from build123d import *

# Parameters (mm, degrees)
ESTRUSIONE_ESTRUSIONE1_DEPTH = 140
FORO_6_5_6_5_1_D             = 6.5
FORO_6_5_6_5_2_AT_2_COUNT    = 2
FORO_6_5_6_5_2_AT_2_PITCH    = 25
TAGLIO_ESTRUSIONE1_REACH     = 158.844
SCHIZZO8_R                   = 1.75
TAGLIO_ESTRUSIONE2_REACH     = 158.844
SCHIZZO9_R                   = 1.75
SCHIZZO9_R_2                 = 7
TAGLIO_ESTRUSIONE4_REACH     = 158.844
SCHIZZO11_R                  = 4
SCHIZZO11_R_2                = 1.75
SMUSSO1_SIZE                 = 3


with BuildPart() as part:
    # Schizzo1 → Estrusione-Estrusione1 (new body)
    with BuildSketch(Plane.XY):
        Polygon((0, 0), (0, 50), (5, 50), (5, 5), (50, 5), (50, 0), align=None)
    extrude(amount=ESTRUSIONE_ESTRUSIONE1_DEPTH)

    # Foro Ø6.5 (6.5)-1 (through all)
    with Locations(Plane(origin=(0, 0, 0), x_dir=(-1, 0, 0), z_dir=(0, -1, 0))):
        with Locations((-17, -132), (-42, -132)):
            Hole(FORO_6_5_6_5_1_D / 2)

    # Schizzo6 → Foro Ø6.5 (6.5)-2 (revolve, cut)
    with BuildSketch(Plane(origin=(0, 42, 132), x_dir=(0, 0, 1), z_dir=(0, 1, 0))):
        Polygon((0, 0), (0, 6.952797012), (3.25, 5), (3.25, 0), align=None)
    foro_6_5_6_5_2 = revolve(axis=Axis((-6.35, 42, 132), (1, 0, 0)), mode=Mode.SUBTRACT)

    # Foro Ø6.5 (6.5)-2 at 2: Foro Ø6.5 (6.5)-2 ×2
    with Locations(*[(0, -i * FORO_6_5_6_5_2_AT_2_PITCH, 0) for i in range(1, FORO_6_5_6_5_2_AT_2_COUNT)]):
        add(foro_6_5_6_5_2, mode=Mode.SUBTRACT)

    # Specchia1: Foro Ø6.5 (6.5)-2 across plane
    add(foro_6_5_6_5_2.mirror(Plane.XY.offset(70)), mode=Mode.SUBTRACT)

    # Specchia1 copy 1 sketch → Specchia1 copy 1 (revolve, cut)
    with BuildSketch(Plane(origin=(0, 17, 8), x_dir=(0, 0, -1), z_dir=(0, 1, 0))):
        Polygon((0, 0), (0, -6.952797012), (3.25, -5), (3.25, 0), align=None)
    revolve(axis=Axis((-6.35, 17, 8), (-1, 0, 0)), mode=Mode.SUBTRACT)

    # Schizzo8 → Taglio-Estrusione1 (cut, up to next)
    with BuildSketch(Plane.XZ, mode=Mode.PRIVATE) as taglio_estrusione1_sk1:
        with Locations((20, 70)):
            Circle(SCHIZZO8_R)
    taglio_estrusione1_tool1 = extrude(taglio_estrusione1_sk1.sketch, amount=-TAGLIO_ESTRUSIONE1_REACH, mode=Mode.PRIVATE) & part.part
    # Schizzo8 → Taglio-Estrusione1 (cut, up to next)
    with BuildSketch(Plane.XZ, mode=Mode.PRIVATE) as taglio_estrusione1_sk2:
        with Locations((20, 90)):
            Circle(SCHIZZO8_R)
    taglio_estrusione1_tool2 = extrude(taglio_estrusione1_sk2.sketch, amount=-TAGLIO_ESTRUSIONE1_REACH, mode=Mode.PRIVATE) & part.part
    # Schizzo8 → Taglio-Estrusione1 (cut, up to next)
    with BuildSketch(Plane.XZ, mode=Mode.PRIVATE) as taglio_estrusione1_sk3:
        with Locations((40, 90)):
            Circle(SCHIZZO8_R)
    taglio_estrusione1_tool3 = extrude(taglio_estrusione1_sk3.sketch, amount=-TAGLIO_ESTRUSIONE1_REACH, mode=Mode.PRIVATE) & part.part
    # Schizzo8 → Taglio-Estrusione1 (cut, up to next)
    with BuildSketch(Plane.XZ, mode=Mode.PRIVATE) as taglio_estrusione1_sk4:
        with Locations((40, 70)):
            Circle(SCHIZZO8_R)
    taglio_estrusione1_tool4 = extrude(taglio_estrusione1_sk4.sketch, amount=-TAGLIO_ESTRUSIONE1_REACH, mode=Mode.PRIVATE) & part.part
    add(taglio_estrusione1_tool1.solids().sort_by_distance((20, 0, 70))[0], mode=Mode.SUBTRACT)
    add(taglio_estrusione1_tool2.solids().sort_by_distance((20, 0, 90))[0], mode=Mode.SUBTRACT)
    add(taglio_estrusione1_tool3.solids().sort_by_distance((40, 0, 90))[0], mode=Mode.SUBTRACT)
    add(taglio_estrusione1_tool4.solids().sort_by_distance((40, 0, 70))[0], mode=Mode.SUBTRACT)

    # Schizzo9 → Taglio-Estrusione2 (cut, up to next)
    with BuildSketch(Plane.ZY, mode=Mode.PRIVATE) as taglio_estrusione2_sk1:
        with Locations((90, 40)):
            Circle(SCHIZZO9_R)
    taglio_estrusione2_tool1 = extrude(taglio_estrusione2_sk1.sketch, amount=-TAGLIO_ESTRUSIONE2_REACH, mode=Mode.PRIVATE) & part.part
    # Schizzo9 → Taglio-Estrusione2 (cut, up to next)
    with BuildSketch(Plane.ZY, mode=Mode.PRIVATE) as taglio_estrusione2_sk2:
        with Locations((110, 40)):
            Circle(SCHIZZO9_R)
    taglio_estrusione2_tool2 = extrude(taglio_estrusione2_sk2.sketch, amount=-TAGLIO_ESTRUSIONE2_REACH, mode=Mode.PRIVATE) & part.part
    # Schizzo9 → Taglio-Estrusione2 (cut, up to next)
    with BuildSketch(Plane.ZY, mode=Mode.PRIVATE) as taglio_estrusione2_sk3:
        with Locations((110, 20)):
            Circle(SCHIZZO9_R)
    taglio_estrusione2_tool3 = extrude(taglio_estrusione2_sk3.sketch, amount=-TAGLIO_ESTRUSIONE2_REACH, mode=Mode.PRIVATE) & part.part
    # Schizzo9 → Taglio-Estrusione2 (cut, up to next)
    with BuildSketch(Plane.ZY, mode=Mode.PRIVATE) as taglio_estrusione2_sk4:
        with Locations((90, 20)):
            Circle(SCHIZZO9_R)
    taglio_estrusione2_tool4 = extrude(taglio_estrusione2_sk4.sketch, amount=-TAGLIO_ESTRUSIONE2_REACH, mode=Mode.PRIVATE) & part.part
    # Schizzo9 → Taglio-Estrusione2 (cut, up to next)
    with BuildSketch(Plane.ZY, mode=Mode.PRIVATE) as taglio_estrusione2_sk5:
        with Locations((100, 30)):
            Circle(SCHIZZO9_R_2)
    taglio_estrusione2_tool5 = extrude(taglio_estrusione2_sk5.sketch, amount=-TAGLIO_ESTRUSIONE2_REACH, mode=Mode.PRIVATE) & part.part
    add(taglio_estrusione2_tool1.solids().sort_by_distance((0, 40, 90))[0], mode=Mode.SUBTRACT)
    add(taglio_estrusione2_tool2.solids().sort_by_distance((0, 40, 110))[0], mode=Mode.SUBTRACT)
    add(taglio_estrusione2_tool3.solids().sort_by_distance((0, 20, 110))[0], mode=Mode.SUBTRACT)
    add(taglio_estrusione2_tool4.solids().sort_by_distance((0, 20, 90))[0], mode=Mode.SUBTRACT)
    add(taglio_estrusione2_tool5.solids().sort_by_distance((0, 30, 100))[0], mode=Mode.SUBTRACT)

    # Schizzo11 → Taglio-Estrusione4 (cut, up to next)
    with BuildSketch(Plane.ZY, mode=Mode.PRIVATE) as taglio_estrusione4_sk1:
        with Locations((43, 26)):
            Circle(SCHIZZO11_R)
    taglio_estrusione4_tool1 = extrude(taglio_estrusione4_sk1.sketch, amount=-TAGLIO_ESTRUSIONE4_REACH, mode=Mode.PRIVATE) & part.part
    # Schizzo11 → Taglio-Estrusione4 (cut, up to next)
    with BuildSketch(Plane.ZY, mode=Mode.PRIVATE) as taglio_estrusione4_sk2:
        with Locations((58.556349186, 41.556349186)):
            Circle(SCHIZZO11_R_2)
    taglio_estrusione4_tool2 = extrude(taglio_estrusione4_sk2.sketch, amount=-TAGLIO_ESTRUSIONE4_REACH, mode=Mode.PRIVATE) & part.part
    # Schizzo11 → Taglio-Estrusione4 (cut, up to next)
    with BuildSketch(Plane.ZY, mode=Mode.PRIVATE) as taglio_estrusione4_sk3:
        with Locations((58.556349186, 10.443650814)):
            Circle(SCHIZZO11_R_2)
    taglio_estrusione4_tool3 = extrude(taglio_estrusione4_sk3.sketch, amount=-TAGLIO_ESTRUSIONE4_REACH, mode=Mode.PRIVATE) & part.part
    # Schizzo11 → Taglio-Estrusione4 (cut, up to next)
    with BuildSketch(Plane.ZY, mode=Mode.PRIVATE) as taglio_estrusione4_sk4:
        with Locations((27.443650814, 10.443650814)):
            Circle(SCHIZZO11_R_2)
    taglio_estrusione4_tool4 = extrude(taglio_estrusione4_sk4.sketch, amount=-TAGLIO_ESTRUSIONE4_REACH, mode=Mode.PRIVATE) & part.part
    # Schizzo11 → Taglio-Estrusione4 (cut, up to next)
    with BuildSketch(Plane.ZY, mode=Mode.PRIVATE) as taglio_estrusione4_sk5:
        with Locations((27.443650814, 41.556349186)):
            Circle(SCHIZZO11_R_2)
    taglio_estrusione4_tool5 = extrude(taglio_estrusione4_sk5.sketch, amount=-TAGLIO_ESTRUSIONE4_REACH, mode=Mode.PRIVATE) & part.part
    add(taglio_estrusione4_tool1.solids().sort_by_distance((0, 26, 43))[0], mode=Mode.SUBTRACT)
    add(taglio_estrusione4_tool2.solids().sort_by_distance((0, 41.556349, 58.556349))[0], mode=Mode.SUBTRACT)
    add(taglio_estrusione4_tool3.solids().sort_by_distance((0, 10.443651, 58.556349))[0], mode=Mode.SUBTRACT)
    add(taglio_estrusione4_tool4.solids().sort_by_distance((0, 10.443651, 27.443651))[0], mode=Mode.SUBTRACT)
    add(taglio_estrusione4_tool5.solids().sort_by_distance((0, 41.556349, 27.443651))[0], mode=Mode.SUBTRACT)

    # Smusso1
    smusso1_edges = [part.edges().sort_by_distance(p)[0] for p in [
        (2.5, 50, 140),
        (2.5, 50, 0),
        (50, 2.5, 140),
        (50, 2.5, 0),
    ]]
    chamfer(smusso1_edges, length=SMUSSO1_SIZE)


solid = part.part
Work out the finished part from the listing and answer in its coordinate system (mm). A direction names the side the tool comes from. Round coordinates to 2 decimals unless told otherwise and drop trailing zeros. Write each loop counter-clockwise with the first axis right and the second up, starting at its lowest first coordinate (ties: lowest second). Pieces come first, ordered by that corner, then holes. Notation, with made-up numbers: (54, 19.25) - (73, 19.25) arc R19 ccw to (73, 55.25) - close; hole circle Ø9 at (62.5, 8). An arc over 180 degrees is marked (long way). Answer in a Markdown table with one row per item. Add a question column.
1. A cutting plane is placed at D-D, the plane x = 36. Determine the outline of the cut face in (y, z).
2. The mould has two halves that part along Z. Classify faces 3 (the cylindrical face through (18.5, 2.535, 134.883)), 4 (the flat face through (13, 4, 0)), 5 (the flat face through (0, 25, 69)): +Z half, -Z half, draft (parallel to the pull), parting line (faces both ways), or undercut.
3. A cutting plane is placed at A-A, the plane z = 104. Determine the outline of the cut face in (x, y).
4. A cutting plane is placed at C-C, the plane z = 78. Determine the outline of the cut face in (x, y), and give its area (3 significant figures).
5. Find the intervals of material crossed by line 1 along Y through (x, z) = (1, 90); line 2 along Y through (x, z) = (3.7, 8), in increasing order. Write a range as from..to.
6. For faces 1 (the flat face through (27, 5, 69)), 2 (the cylindrical face through (2.465, 45.173, 8.705)), determine the directions among +Z, -Z, +X, -X, +Y, -Y from which every point of the face is accessible in a straight line to the end or side of a thin tool.
7. A cutting plane is placed at B-B, the plane y = 26. Determine the outline of the cut face in (x, z), and give its area (3 significant figures).
8. Given pin 1 (6 mm diameter, centred on x = 17, z = 132, fed in from -Y); pin 2 (18 mm diameter, centred on y = 30, z = 100, fed in from +X); pin 3 (4 mm diameter, centred on y = 20, z = 110, fed in from -X); pin 4 (4 mm diameter, centred on x = 40, z = 90, fed in from +Y), each flat-ended and moving along its own axis, determine where each tip first touches the part or whether it passes through.
Worked out:
| question | item | result |
|---|---|---|
| 1 | outline | (0, 0) - (5, 0) - (5, 140) - (0, 140) - close |
| 2 | face 3 | undercut |
| 2 | face 4 | -Z half |
| 2 | face 5 | draft |
| 3 | outline | (0, 0) - (50, 0) - (50, 5) - (5, 5) - (5, 24.26) - (0, 24.26) - close; (0, 35.74) - (5, 35.74) - (5, 50) - (0, 50) - close |
| 4 | outline | (0, 0) - (50, 0) - (50, 5) - (5, 5) - (5, 50) - (0, 50) - close |
| 4 | area | 475 mm^2 |
| 5 | line 1 | 0..18.25, 21.75..38.25, 41.75..50 |
| 5 | line 2 | 0..13.75, 20.25..38.75, 45.25..50 |
| 6 | face 1 | +Z, -Z, +X, +Y |
| 6 | face 2 | +X, -X |
| 7 | outline | (0, 0) - (5, 0) - (5, 39) - (0, 39) - close; (0, 47) - (5, 47) - (5, 94.26) - (0, 94.26) - close; (0, 105.74) - (5, 105.74) - (5, 140) - (0, 140) - close |
| 7 | area | 603 mm^2 |
| 8 | pin 1 | through |
| 8 | pin 2 | x = 5 |
| 8 | pin 3 | x = 0 |
| 8 | pin 4 | y = 5 |
